```python
from build123d import *

# Parameters (mm, degrees)
F0_W     = 260
F0_H     = 184
F0_W_2   = 256
F0_H_2   = 180
F1_DEPTH = 14
F0_W_3   = 208.88
F0_H_3   = 167.12
F2_DEPTH = 4
F0_W_4   = 196.608
F0_H_4   = 147.456
F3_DEPTH = 2


with BuildPart() as f1:
    # F0 (on Front) → F1 (new body)
    with BuildSketch(Plane.XZ):
        with Locations((19.391128, 2.061408)):
            Rectangle(F0_W, F0_H)
        with Locations((19.391128, 2.061408)):
            Rectangle(F0_W_2, F0_H_2, mode=Mode.SUBTRACT)
    extrude(amount=-F1_DEPTH)

    # F0 (on Front) → F2 (join)
    with BuildSketch(Plane.XZ):
        with Locations((19.391128, 2.061408)):
            Rectangle(F0_W_2, F0_H_2)
        Rectangle(F0_W_3, F0_H_3, mode=Mode.SUBTRACT)
    extrude(amount=-F2_DEPTH)

    # F0 (on Front) → F3 (join)
    with BuildSketch(Plane.XZ):
        Rectangle(F0_W_3, F0_H_3)
        Rectangle(F0_W_4, F0_H_4, mode=Mode.SUBTRACT)
    extrude(amount=-F3_DEPTH)


solid = f1.part
```
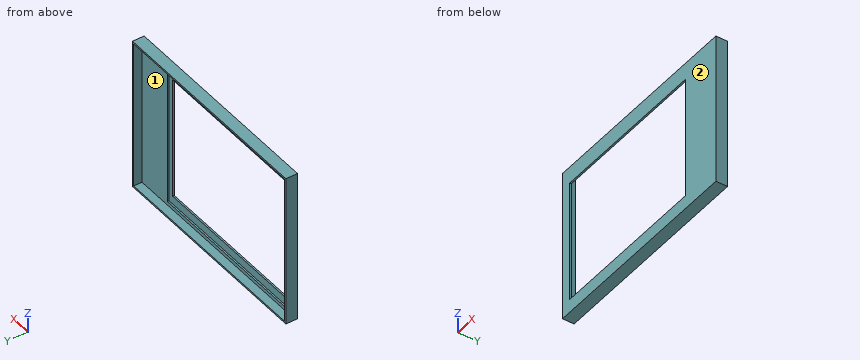
Work out the finished part from the listing and answer in its coordinate system (mm). Face numbers are marked on the shaded views. Give positions to 0.01 mm unless a question says otherwise; leave off trailing zeros. Write each loop counter-clockwise with the first axis right and the second up, starting at its lowest first coordinate (ties: lowest second). Pieces come first, ordered by that corner, then holes. Notation, with made-up numbers: (60.25, -35.75) -> (86.25, -35.75) arc R22 cw to (86.25, -25.75) -> close; hole circle Ø9 at (75.5, 22). An arc over 180 degrees is marked (long way). Write item = value, one per line.
Q1. Section C-C on y = 10 is taken. Determine the outline of the cut face in (x, z).
Computed values:
outline = (-110.61, -89.94) -> (149.39, -89.94) -> (149.39, 94.06) -> (-110.61, 94.06) -> close; hole (-108.61, -87.94) -> (147.39, -87.94) -> (147.39, 92.06) -> (-108.61, 92.06) -> close
Q2. For a pull along Z with two mould halves and no side action, classify the marked faces 1 and 2 as pulls with the +Z half, pulls with the -Z half, needs draft (parallel to the pull), parting line crosses it, or undercut.
Computed values:
face_1 = undercut
face_2 = needs draft
Q3. Section B-B on z = -28 is taken. Determine the outline of the cut face in (x, y).
Computed values:
outline = (-110.61, 0) -> (-98.3, 0) -> (-98.3, 2) -> (-104.44, 2) -> (-104.44, 4) -> (-108.61, 4) -> (-108.61, 14) -> (-110.61, 14) -> close; (98.3, 0) -> (149.39, 0) -> (149.39, 14) -> (147.39, 14) -> (147.39, 4) -> (104.44, 4) -> (104.44, 2) -> (98.3, 2) -> close
Q4. Consider line 1 along X through (y, z) = (11, -63); line 2 along Z through (x, y) = (104.5, 12.25); line 3 along Z through (x, y) = (36, 1.5). Determine where each line is inside the solid, lowest interval first.
Computed values:
line_1 = -110.61 to -108.61, 147.39 to 149.39
line_2 = -89.94 to -87.94, 92.06 to 94.06
line_3 = -89.94 to -73.73, 73.73 to 94.06
Q5. Section A-A on x = -47 is taken. Determine the outline of the cut face in (y, z), and give its area (3 significant figures).
Computed values:
outline = (0, -89.94) -> (14, -89.94) -> (14, -87.94) -> (4, -87.94) -> (4, -83.56) -> (2, -83.56) -> (2, -73.73) -> (0, -73.73) -> close; (0, 73.73) -> (2, 73.73) -> (2, 83.56) -> (4, 83.56) -> (4, 92.06) -> (14, 92.06) -> (14, 94.06) -> (0, 94.06) -> close
area = 147 mm^2
